from build123d import *

# Parameters (mm, degrees)
SKETCH1_W           = 63.246
SKETCH1_H           = 65.786
BOSS_EXTRUDE1_DEPTH = 3.302
FILLET2_R           = 5.08
SKETCH2_R           = 14.732
SKETCH2_R_2         = 3.81
CUT_EXTRUDE1_DEPTH  = 9.652


with BuildPart() as part:
    # Sketch1 → Boss-Extrude1 (new body)
    with BuildSketch(Plane(origin=(0, 0, 0), x_dir=(1, 0, 0), z_dir=(0, 1, 0))):
        with Locations((-31.623, 32.893)):
            Rectangle(SKETCH1_W, SKETCH1_H)
    extrude(amount=BOSS_EXTRUDE1_DEPTH)

    # Fillet2
    fillet2_edges = [part.edges().sort_by_distance(p)[0] for p in [
        (0, 1.651, 0),
        (-63.246, 1.651, 0),
        (-63.246, 1.651, -65.786),
        (0, 1.651, -65.786),
    ]]
    fillet(fillet2_edges, radius=FILLET2_R)

    # Sketch2 → Cut-Extrude1 (cut)
    with BuildSketch(Plane(origin=(0, 3.302, 0), x_dir=(1, 0, 0), z_dir=(0, 1, 0))):
        with Locations(Location((-30.988, 40.64, 0), (0, 0, 270))):
            Circle(SKETCH2_R)
        with Locations(Location((-53.086, 49.53, 0), (0, 0, 270))):
            Circle(SKETCH2_R_2)
        with Locations(Location((-9.398, 31.496, 0), (0, 0, 270))):
            Circle(SKETCH2_R_2)
    extrude(amount=-CUT_EXTRUDE1_DEPTH, mode=Mode.SUBTRACT)


solid = part.part
Source: CAD feature listing. Evaluate the final solid. Frame: model axes, mm. Round coordinates to 2 decimals unless told otherwise and drop trailing zeros. Loops run counter-clockwise (first coordinate to the right, second up) from the corner with the lowest first, then second, coordinate; pieces in that order, holes last. Notation, with made-up numbers: (-12.75, 53) -> (14.25, 53) arc R32 cw to (14.25, 83) -> close; hole circle Ø6 at (22, 15.25). An arc over 180 degrees is marked (long way). Answer as a JSON object with one key per item and string values. Group by question number.
Q1. Section query D-D (y = 1.75). Output: boundary loops of the cut face in (x, z), plus the area to 3 significant figures.
Q2. Section query B-B (x = -34.5). Output: boundary loops of the cut face in (y, z), plus the area to 3 significant figures.
Q3. Section query C-C (z = -49.53). Output: boundary loops of the cut face in (x, y).
Q4. Ray query, line 1 (X direction, y = 0.85, z = -47); line 2 (X direction, y = 1.3, z = -53); line 3 (X direction, y = 1.55, z = -40.64). Return the intervals inside material, ascending. Write a range as from..to.
Q5. Mould query, pull axis Z, two halves, no side actions, for faces 1 (the flat face through (0, 2, -33)), 2 (the cylindrical face through (-39.95, 1.67, -52.33)), 3 (the cylindrical face through (-1.45, 1.67, -64.26)), 4 (the flat face through (-32, 2, 0)). Classes: pulls with the +Z half, pulls with the -Z half, needs draft (parallel to the pull), parting line crosses it, or undercut.
Q6. Section query A-A (z = -40.64). Output: boundary loops of the cut face in (x, y).
Completed:
{
 "1": {"outline": "(-63.25, -60.71) arc R5.08 ccw to (-58.17, -65.79) -> (-5.08, -65.79) arc R5.08 ccw to (0, -60.71) -> (0, -5.08) arc R5.08 ccw to (-5.08, 0) -> (-58.17, 0) arc R5.08 ccw to (-63.25, -5.08) -> close; hole circle Ø7.62 at (-53.09, -49.53); hole circle Ø29.46 at (-30.99, -40.64); hole circle Ø7.62 at (-9.4, -31.5)", "area": "3,370 mm²"},
 "2": {"outline": "(0, -65.79) -> (3.3, -65.79) -> (3.3, -54.95) -> (0, -54.95) -> close; (0, -26.33) -> (3.3, -26.33) -> (3.3, 0) -> (0, 0) -> close", "area": "123 mm²"},
 "3": {"outline": "(-63.25, 0) -> (-56.9, 0) -> (-56.9, 3.3) -> (-63.25, 3.3) -> close; (-49.28, 0) -> (-42.74, 0) -> (-42.74, 3.3) -> (-49.28, 3.3) -> close; (-19.24, 0) -> (0, 0) -> (0, 3.3) -> (-19.24, 3.3) -> close"},
 "4": {"line 1": "-63.25..-55.93, -50.24..-44.28, -17.7..0", "line 2": "-63.25..-54.66, -51.51..-39, -22.97..0", "line 3": "-63.25..-45.72, -16.26..0"},
 "5": {"face 1": "needs draft", "face 2": "undercut", "face 3": "pulls with the -Z half", "face 4": "pulls with the +Z half"},
 "6": {"outline": "(-63.25, 0) -> (-45.72, 0) -> (-45.72, 3.3) -> (-63.25, 3.3) -> close; (-16.26, 0) -> (0, 0) -> (0, 3.3) -> (-16.26, 3.3) -> close"}
}
